Read the model definition and answer for the solid it produces. Units are mm, in the model's axes. A direction names the side the tool comes from. Round coordinates to 2 decimals unless told otherwise and drop trailing zeros. Write each loop counter-clockwise with the first axis right and the second up, starting at its lowest first coordinate (ties: lowest second). Pieces come first, ordered by that corner, then holes. Notation, with made-up numbers: (61.25, -21.5) -> (79.25, -21.5) arc R32 cw to (79.25, 14.5) -> close; hole circle Ø8 at (12.5, -26). An arc over 180 degrees is marked (long way). Return JSON: item names as keys, results as strings. Group by question number.
(1) A cutting plane is placed at B-B on x = 56.5. State how many separate pieces and enclosed holes the cut face has, then the cut area to 3 significant figures.
(2) For faces 4 (the flat face through (22, -7, -59)), 5 (the flat face through (32, 5, 0)), 6 (the flat face through (20, 5, -44)), 7 (the cylindrical face through (41.6, 4.93, -19.43)), determine the directions among +Z, -Z, +X, -X, +Y, -Y from which every point of the face is accessible in a straight line to the end or side of a thin tool.
(3) Straight lines are drawn through the part: line 1 (X direction, y = 6.5, z = -56.5); line 2 (X direction, y = 2.25, z = -32.5); line 3 (Z direction, x = 8.5, y = 8.5). For each, find the intervals that lie inside material, in ascending order.
(4) A cutting plane is placed at D-D on y = -5.5. Give the vertices of the cut face in (x, z).
(5) The mould has two halves that part along Z. Classify faces 1 (the cylindrical face through (-4, -2, -63)), 2 (the flat face through (41, 5, -11)), 3 (the flat face through (58, -7, -22)): released by +Z, released by -Z, zero draft, split by the parting line, or undercut.
(6) A cutting plane is placed at A-A on z = -32.5. Give the vertices of the cut face in (x, y).
(7) Given pin 1 (10.5 mm diameter, centred on y = -10.5, z = -58, fed in from +X); pin 2 (3 mm diameter, centred on x = 20, z = -32.5, fed in from -Y); pin 3 (5 mm diameter, centred on y = -8, z = -29, fed in from +X); pin 4 (2 mm diameter, centred on x = 50.5, z = -22.5, fed in from -Y), each flat-ended and moving along its own axis, determine where each tip first touches the part or whether it passes through.
```python
from build123d import *

# Parameters (mm, degrees)
SKETCH1_W                = 65
SKETCH1_H                = 65
BOSS_EXTRUDE2_DEPTH      = 10
SKETCH6_R                = 1.35
CUT_EXTRUDE3_DEPTH       = 93.466210045
SKETCH7_R                = 2.6
SKETCH7_W                = 20
SKETCH7_H                = 7
SKETCH7_W_2              = 7
SKETCH7_H_2              = 20
CUT_EXTRUDE4_DEPTH       = 93.466210045
SKETCH9_W                = 15
SKETCH9_H                = 6
SKETCH9_W_2              = 6
SKETCH9_H_2              = 15
BOSS_EXTRUDE5_DEPTH      = 15
FILLET4_R                = 2
FILLET5_R                = 1
FILLET6_R                = 1
BOSS_EXTRUDE6_DEPTH      = 15
BOSS_EXTRUDE6_DEPTH_BACK = 10
SKETCH10_W               = 17
SKETCH10_H               = 5
SKETCH10_W_2             = 5
SKETCH10_H_2             = 17
FILLET7_R                = 5
FILLET8_R                = 1
SKETCH11_R               = 2.6
CUT_EXTRUDE5_DEPTH       = 96.262794579


with BuildPart() as part:
    # Sketch1 → Boss-Extrude2 (new body)
    with BuildSketch(Plane(origin=(0, 0, 0), x_dir=(1, 0, 0), z_dir=(0, 1, 0))):
        with Locations((32.5, 32.5)):
            Rectangle(SKETCH1_W, SKETCH1_H)
    extrude(amount=BOSS_EXTRUDE2_DEPTH)

    # Sketch6 → Cut-Extrude3 (cut, through all)
    with BuildSketch(Plane(origin=(0, 10, 0), x_dir=(1, 0, 0), z_dir=(0, 1, 0))):
        with Locations(Location((56.5, 56.5, 0), (0, 0, 270))):
            Circle(SKETCH6_R)
        with Locations(Location((32.5, 56.5, 0), (0, 0, 270))):
            Circle(SKETCH6_R)
        with Locations(Location((32.5, 32.5, 0), (0, 0, 270))):
            Circle(SKETCH6_R)
        with Locations(Location((56.5, 32.5, 0), (0, 0, 270))):
            Circle(SKETCH6_R)
    extrude(amount=-CUT_EXTRUDE3_DEPTH, mode=Mode.SUBTRACT)

    # Sketch7 → Cut-Extrude4 (cut, through all)
    with BuildSketch(Plane(origin=(0, 10, 0), x_dir=(1, 0, 0), z_dir=(0, 1, 0))):
        with Locations(Location((10, 32.5, 0), (0, 0, 270))):
            Circle(SKETCH7_R)
        with Locations(Location((10, 56.5, 0), (0, 0, 270))):
            Circle(SKETCH7_R)
        with Locations(Location((32.5, 10, 0), (0, 0, 270))):
            Circle(SKETCH7_R)
        with Locations(Location((56.5, 10, 0), (0, 0, 270))):
            Circle(SKETCH7_R)
        with Locations((10, 44.5)):
            Rectangle(SKETCH7_W, SKETCH7_H)
        with Locations((44.5, 10)):
            Rectangle(SKETCH7_W_2, SKETCH7_H_2)
        Polygon((0, 24), (20, 24), (20, 20), (24, 20), (24, 0), (20, 0), (0, 0), (0, 20), align=None)
    extrude(amount=-CUT_EXTRUDE4_DEPTH, mode=Mode.SUBTRACT)

    # Sketch9 → Boss-Extrude5 (add)
    with BuildSketch(Plane.XZ):
        with Locations((57.5, -25)):
            Rectangle(SKETCH9_W, SKETCH9_H)
        with Locations((25, -57.5)):
            Rectangle(SKETCH9_W_2, SKETCH9_H_2)
    extrude(amount=BOSS_EXTRUDE5_DEPTH)

    # Fillet4
    fillet4_edges = [part.edges().sort_by_distance(p)[0] for p in [
        (50, -7.5, -22),
        (50, -7.5, -28),
        (22, -7.5, -50),
        (28, -7.5, -50),
        (41, 5, -20),
        (48, 5, -20),
        (20, 5, -48),
        (20, 5, -41),
    ]]
    fillet(fillet4_edges, radius=FILLET4_R)

    # Fillet5
    fillet5_edges = [part.edges().sort_by_distance(p)[0] for p in [
        (58.5, 0, -22),
        (28, 0, -58.5),
        (22, 0, -58.5),
        (25, 0, -50),
        (58.5, 0, -28),
        (50, 0, -25),
        (22.585786438, 0, -50.585786438),
        (27.414213562, 0, -50.585786438),
        (50.585786438, 0, -27.414213562),
        (50.585786438, 0, -22.585786438),
    ]]
    fillet(fillet5_edges, radius=FILLET5_R)

    # Fillet6
    fillet6_edges = [part.edges().sort_by_distance(p)[0] for p in [
        (65, -15, -25),
        (58.5, -15, -22),
        (25, -15, -65),
        (28, -15, -58.5),
        (22, -15, -58.5),
        (25, -15, -50),
        (27.414213562, -15, -50.585786438),
        (22.585786438, -15, -50.585786438),
        (58.5, -15, -28),
        (50, -15, -25),
        (50.585786438, -15, -22.585786438),
        (50.585786438, -15, -27.414213562),
    ]]
    fillet(fillet6_edges, radius=FILLET6_R)

    # Sketch10 → Boss-Extrude6 (add, two sides: drawn at the far end of the back side and taken through both)
    with BuildSketch(Plane.XZ.offset(-BOSS_EXTRUDE6_DEPTH_BACK)):
        with Locations((56.5, 2.5)):
            Rectangle(SKETCH10_W, SKETCH10_H)
        with Locations((-2.5, -56.5)):
            Rectangle(SKETCH10_W_2, SKETCH10_H_2)
    extrude(amount=BOSS_EXTRUDE6_DEPTH + BOSS_EXTRUDE6_DEPTH_BACK)

    # Fillet7
    # the kernel refuses this fillet: 5 mm, written as the material it takes off along each edge
    with BuildSketch(Plane(origin=(65, -12.5, -65), x_dir=(-1, 0, 0), z_dir=(0, 1, 0)), Plane(origin=(41, 22.5, 0), x_dir=(-1, 0, 0), z_dir=(0, -1, 0)), Plane(origin=(24, 22.5, 0), x_dir=(0, 0, -1), z_dir=(0, -1, 0)), Plane(origin=(0, 22.5, -24), x_dir=(0, 0, -1), z_dir=(0, -1, 0)), Plane(origin=(0, 22.5, -41), x_dir=(1, 0, 0), z_dir=(0, -1, 0))) as fillet7_piece_1:
        with BuildLine():
            CenterArc((FILLET7_R, FILLET7_R), FILLET7_R, 180, 90)
            Line((0, FILLET7_R), (0, 0))
            Line((0, 0), (FILLET7_R, 0))
        make_face()
    extrude(amount=35, mode=Mode.SUBTRACT)
    with BuildSketch(Plane(origin=(65, 22.5, 5), x_dir=(-1, 0, 0), z_dir=(0, -1, 0)), Plane(origin=(-5, 22.5, -65), x_dir=(1, 0, 0), z_dir=(0, -1, 0))) as fillet7_piece_2:
        with BuildLine():
            CenterArc((FILLET7_R, FILLET7_R), FILLET7_R, 180, 90)
            Line((0, FILLET7_R), (0, 0))
            Line((0, 0), (FILLET7_R, 0))
        make_face()
    extrude(amount=50, mode=Mode.SUBTRACT)
    with BuildSketch(Plane(origin=(48, -27.5, 5), x_dir=(0, 0, -1), z_dir=(0, 1, 0)), Plane(origin=(-5, 22.5, -48), x_dir=(1, 0, 0), z_dir=(0, -1, 0))) as fillet7_piece_3:
        with BuildLine():
            CenterArc((FILLET7_R, -FILLET7_R), FILLET7_R, 90, 90)
            Line((0, -FILLET7_R), (0, 0))
            Line((0, 0), (FILLET7_R, 0))
        make_face()
    extrude(amount=50, mode=Mode.SUBTRACT)
    with BuildSketch(Plane(origin=(20, 20, -20), x_dir=(0, 0, -1), z_dir=(0, -1, 0))) as fillet7_piece_4:
        with BuildLine():
            CenterArc((4.915475947, 4.915475947), FILLET7_R, 190.550098012, 68.899803976)
            Line((0, 4), (0, 0))
            Line((0, 0), (4, 0))
        make_face()
    extrude(amount=30, mode=Mode.SUBTRACT)

    # Fillet8
    fillet8_edges = [part.edges().sort_by_distance(p)[0] for p in [
        (56.5, -15, 0),
        (0, -15, -56.5),
        (56.5, -15, 5),
        (49.464466094, -15, 3.535533906),
        (63.535533906, -15, 3.535533906),
        (-5, -15, -56.5),
        (-3.535533906, -15, -63.535533906),
        (-3.535533906, -15, -49.464466094),
        (56.5, 0, 0),
        (0, 0, -56.5),
    ]]
    fillet(fillet8_edges, radius=FILLET8_R)

    # Sketch11 → Cut-Extrude5 (cut, through all)
    with BuildSketch(Plane(origin=(0, 10, 0), x_dir=(1, 0, 0), z_dir=(0, 1, 0))):
        with Locations(Location((20, 32.5, 0), (0, 0, 270))):
            Circle(SKETCH11_R)
    extrude(amount=-CUT_EXTRUDE5_DEPTH, mode=Mode.SUBTRACT)


solid = part.part
```
Checks:
{
 "1": {"separate pieces": "4", "enclosed holes": "0", "area": "759 mm^2"},
 "2": {"face 4": "+Z, -Z, -Y", "face 5": "+Z, -X, +Y, -Y", "face 6": "-X, +Y, -Y", "face 7": "+Z, +Y, -Y"},
 "3": {"line 1": "x = -5 to 7.4, 12.6 to 31.15, 33.85 to 55.15, 57.85 to 65", "line 2": "x = 0 to 7.4, 12.6 to 17.4, 22.6 to 31.15, 33.85 to 55.15, 57.85 to 65", "line 3": "z = -65 to -58.62, -54.38 to -48, -41 to -34.62, -30.38 to -24"},
 "4": {"outline": "(-5, -60) arc R5 ccw to (0, -65) -> (0, -48) arc R5 ccw to (-5, -53) -> close; (22, -65) -> (28, -65) -> (28, -52) arc R2 ccw to (26, -50) -> (24, -50) arc R2 ccw to (22, -52) -> close; (48, 0) -> (65, 0) arc R5 ccw to (60, 5) -> (53, 5) arc R5 ccw to start; (50, -26) arc R2 ccw to (52, -28) -> (65, -28) -> (65, -22) -> (52, -22) arc R2 ccw to (50, -24) -> close"},
 "5": {"face 1": "released by -Z", "face 2": "zero draft", "face 3": "undercut"},
 "6": {"outline": "(0, 0) -> (7.4, 0) -> (7.4, 10) -> (0, 10) -> close; (12.6, 0) -> (17.4, 0) -> (17.4, 10) -> (12.6, 10) -> close; (22.6, 0) -> (31.15, 0) -> (31.15, 10) -> (22.6, 10) -> close; (33.85, 0) -> (55.15, 0) -> (55.15, 10) -> (33.85, 10) -> close; (57.85, 0) -> (65, 0) -> (65, 10) -> (57.85, 10) -> close"},
 "7": {"pin 1": "stops at x = 28", "pin 2": "passes through", "pin 3": "stops at x = 65", "pin 4": "stops at y = -14.99"}
}
